Verification items for the finished model (mm, model axes). A direction names the side the tool comes from. Give positions to 0.01 mm unless a question says otherwise; leave off trailing zeros. Loops run counter-clockwise (first coordinate to the right, second up) from the corner with the lowest first, then second, coordinate; pieces in that order, holes last. Notation, with made-up numbers: M 66,85.5 L 99,85.5 A19 ccw 99,91.5 Z; hole C 70,-2.75 d3. An arc over 180 degrees is marked long. Answer in a Markdown table with one row per item.
```python
from build123d import *

# Parameters (mm, degrees)
SKETCH_1_R      = 0.3
EXTRUDE_1_DEPTH = 1


with BuildPart() as part:
    # 草图1 → 凸台-拉伸1 (new body)
    with BuildSketch(Plane.XY):
        with BuildLine():
            Line((-5, 0), (-33.91366459, -8))
            ThreePointArc((-33.91366459, -8), (-34.610786743, -9.230455486), (-33.380331256, -9.927577639))
            ThreePointArc((-33.380331256, -9.927577639), (-19.285084677, -6.509330991), (-5, -4))
            Line((-5, -4), (5, -4))
            Line((5, -4), (33.646997923, -9.96378882))
            ThreePointArc((33.646997923, -9.96378882), (34.637903776, -9.098345834), (33.91366459, -8))
            Line((33.91366459, -8), (5, 0))
            Line((5, 0), (-5, 0))
        make_face()
        with Locations((-33.646997923, -8.96378882)):
            Circle(SKETCH_1_R, mode=Mode.SUBTRACT)
        with Locations((5, -2)):
            Circle(SKETCH_1_R, mode=Mode.SUBTRACT)
        with Locations((33.646997923, -8.96378882)):
            Circle(SKETCH_1_R, mode=Mode.SUBTRACT)
    extrude(amount=EXTRUDE_1_DEPTH)


solid = part.part
```
Item 1: Sectioned sample at D-D (x = -19). Record the cut outline in (y, z), and give its area (3 significant figures).
Reported:
| item | result |
|---|---|
| outline | M -6.45,0 L -3.87,0 L -3.87,1 L -6.45,1 Z |
| area | 2.58 mm^2 |
Item 2: Tool access check on faces 4 (the flat face through (19.12, -6.94, 0.49)), 5 (the flat face through (0, -3, 1)). Record the directions out of +Z, -Z, +X, -X, +Y, -Y that give a thin tool (end or side, any length) a straight path to the whole face; none if there is none.
Reported:
| item | result |
|---|---|
| face 4 | +Z, -Z, -Y |
| face 5 | +Z, +X, -X, +Y, -Y |
Item 3: Sectioned sample at C-C (x = -3). Record the cut outline in (y, z).
Reported:
| item | result |
|---|---|
| outline | M -4,0 L 0,0 L 0,1 L -4,1 Z |
Item 4: Scan lines: L1, parallel to Y at x = -1, z = 0.5; L2, parallel to Y at x = -21, z = 0.9. Record each from-to range of solid material in increasing order. Write a range as [from, to].
Reported:
| item | result |
|---|---|
| L1 | y = [-4, 0] |
| L2 | y = [-6.87, -4.43] |
Item 5: Sectioned sample at A-A (y = -5.25). Record the cut outline in (x, z).
Reported:
| item | result |
|---|---|
| outline | M -23.97,0 L -12.78,0 L -12.78,1 L -23.97,1 Z; M 11,0 L 23.97,0 L 23.97,1 L 11,1 Z |
Item 6: Go/stop test with a flat-tipped pin: pin 1 (1.5 mm diameter, centred on x = 7, y = -5.5, fed in from +Z). Record where the tip stops, or that it passes through.
Reported:
| item | result |
|---|---|
| pin 1 | passes through |
Item 7: Release check for a two-part mould opening along X. For faces 1 (the flat face through (-19.254, -3.944, 0.493)), 2 (the cylindrical face through (-19.48, -6.55, 0.49)), 3 (the flat face through (0, -3, 0)) record: released by +X, released by -X, zero draft, split by the parting line, or undercut.
Reported:
| item | result |
|---|---|
| face 1 | released by -X |
| face 2 | undercut |
| face 3 | zero draft |
Item 8: Sectioned sample at B-B (z = 0.15). Record the cut outline in (x, y).
Reported:
| item | result |
|---|---|
| outline | M -33.91,-8 A1 ccw -33.38,-9.93 A226.55 cw -5,-4 L 5,-4 L 33.65,-9.96 A1 ccw 33.91,-8 L 5,0 L -5,0 Z; hole C -33.65,-8.96 d0.6; hole C 5,-2 d0.6; hole C 33.65,-8.96 d0.6 |
